Here's how the part is built. I have some questions about the finished solid (model axes, mm). Face numbers are marked on the shaded views. A direction names the side the tool comes from. Give positions to 0.01 mm unless a question says otherwise; leave off trailing zeros. Loops run counter-clockwise (first coordinate to the right, second up) from the corner with the lowest first, then second, coordinate; pieces in that order, holes last. Notation, with made-up numbers: (-10.75, -37) -> (38.25, -37) arc R28 cw to (38.25, 2) -> close; hole circle Ø3 at (71, 76.25). An arc over 180 degrees is marked (long way). Answer in a Markdown table with one row per item. Add a question column.
Item 1: If I drill on line 1 (Z direction, x = 0.1, y = 0); line 2 (Y direction, x = -0.95, z = 0.65), over which ranges is the centre line in solid material (lowest first)?
Item 2: We'd pull the mould along Z, two halves only. Please class the marked faces 1 and 2: released by +Z, released by -Z, zero draft, split by the parting line, or undercut.
Item 3: Which directions (+Z, -Z, +X, -X, +Y, -Y) give clear straight access to the entire face, cutting with the end or side of a thin tool? Please do the marked faces 3 and 4.
Item 4: If we section it at B-B (y = 19.5): Write out the boundary of the cut face in (x, z).
Item 5: For P1, Ø1.3, axis at x = 0, y = -1.5, coming from the +Z side; P2, Ø0.6, axis at x = 0, y = -1, coming from the -Z side, each with a flat end and sliding along its axis, tell me the tip position at first contact or that it passes through.
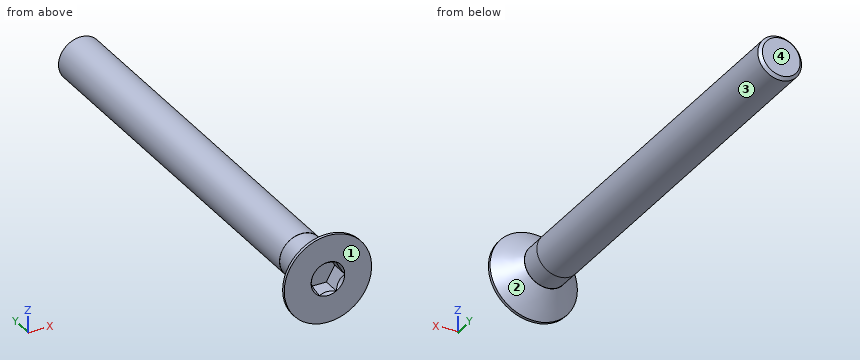
```python
from build123d import *

# Parameters (mm, degrees)
CHAMFER1_SIZE   = 0.2
HEX_DEPTH_DEPTH = 1.2
SKETCH4_R       = 1
SKETCH3_R       = 1.154700538


with BuildPart() as part:
    # Sketch1 → Revolve1 (revolve)
    with BuildSketch(Plane.XY):
        Polygon((0, -1.873883868), (-3, -1.873883868), (-3, -1.673883868), (-1.5, -0.173883868), (-1.49, -0.173883868), (-1.49, 1.326116132), (-1.5, 1.326116132), (-1.5, 28.126116132), (0, 28.126116132), align=None)
    revolve(axis=Axis((0, 0, 0), (0, 1, 0)))

    # Chamfer1
    chamfer1_edges = [part.edges().sort_by_distance(p)[0] for p in [
        (1.5, 28.126116132, 0),
    ]]
    chamfer(chamfer1_edges, length=CHAMFER1_SIZE)

    # Sketch2 → hex depth (cut)
    with BuildSketch(Plane.XZ.offset(1.873883868)):
        Polygon((1.154700538, 0), (0.577350269, 1), (-0.577350269, 1), (-1.154700538, 0), (-0.577350269, -1), (0.577350269, -1), align=None)
    extrude(amount=-HEX_DEPTH_DEPTH, mode=Mode.SUBTRACT)

    # Sketch4 → hex corner cut section 0
    with BuildSketch(Plane(origin=(0, -1.673883868, 0), x_dir=(1, 0, 0), z_dir=(0, 1, 0))):
        Circle(SKETCH4_R)
    # Sketch3 → hex corner cut section 1
    with BuildSketch(Plane.XZ.offset(1.873883868)):
        Circle(SKETCH3_R)
    loft(mode=Mode.SUBTRACT)


solid = part.part
```
Recorded:
| question | item | result |
|---|---|---|
| 1 | line 1 | z = -1.49 to 1.49 |
| 1 | line 2 | y = -1.87 to 28.13 |
| 2 | face 1 | zero draft |
| 2 | face 2 | split by the parting line |
| 3 | face 3 | +Y |
| 3 | face 4 | +Z, -Z, +X, -X, +Y |
| 4 | outline | circle Ø3 at (0, 0) |
| 5 | P1 | stops at z = 3 |
| 5 | P2 | stops at z = -2.63 |
